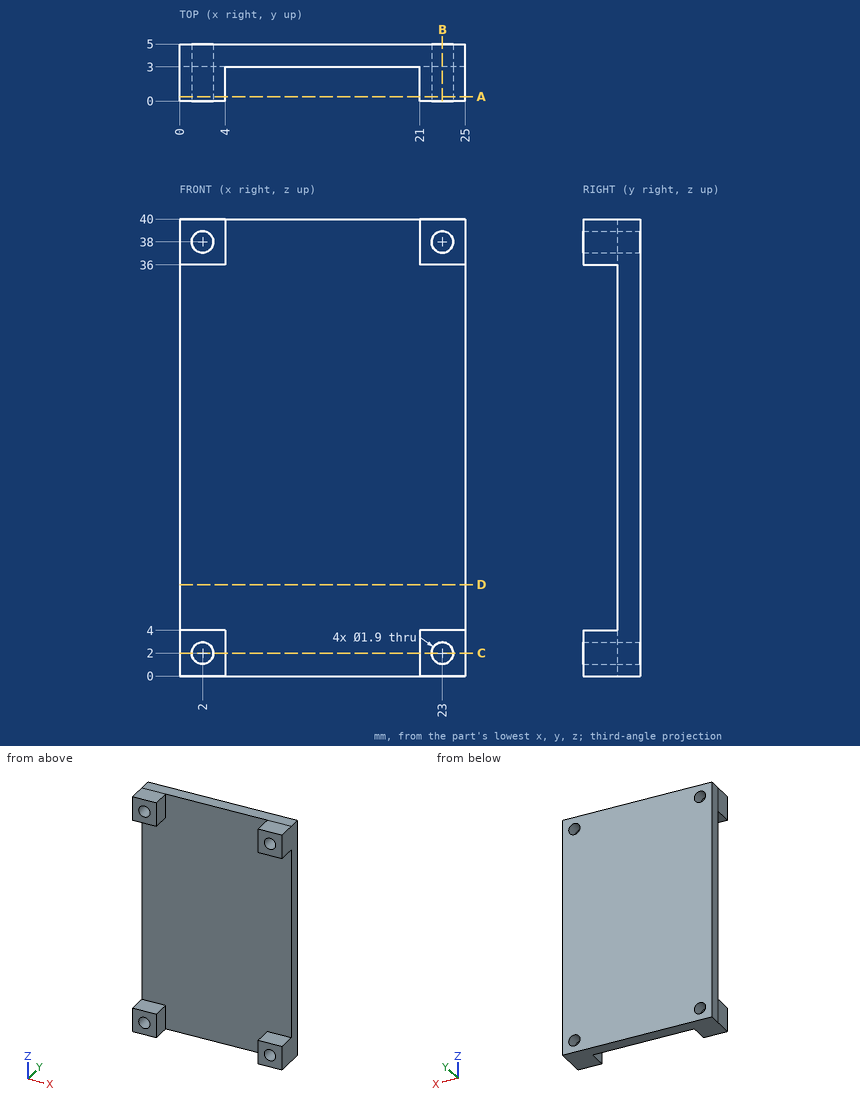
Job drawing, mm, ordinate dimensions from the low corner. One solid piece. Coordinates: 2 decimals unless noted, no trailing zeros. Order: outer loops, then holes, each group sorted by start corner. A loop starts at its lowest first (then second) coordinate and runs counter-clockwise, first axis right, second up. Notation, with made-up numbers: M -36.75,-16.75 L 0.25,-16.75 A24 cw 0.25,5.25 Z; hole C 53,49.5 d10. An arc over 180 degrees is marked long. One line per question, with ' | ' between items.
Q1. Pin check, flat tip, straight feed: P1, Ø7.5, axis at x = 10, z = 17, coming from the -Y side. Stop position of the tip, or through.
A:
P1: stops at y = 3
Q2. Slice it at B-B (x = 23). Give the cut face in (y, z), and give its area (3 significant figures).
A:
outline: M 0,0 L 5,0 L 5,1.05 L 0,1.05 Z; M 0,2.95 L 5,2.95 L 5,37.05 L 0,37.05 L 0,36 L 3,36 L 3,4 L 0,4 Z; M 0,38.95 L 5,38.95 L 5,40 L 0,40 Z | area: 85.0 mm^2
Q3. Slice it at D-D (z = 8). Give the cut face in (x, y).
A:
outline: M 0,3 L 25,3 L 25,5 L 0,5 Z
Q4. Drill centre lines: line 1 (X direction, y = 3.5, z = 2); line 2 (Z direction, x = 23, y = 0.9); line 3 (Y direction, x = 8.75, z = 11). Where is each one in solid material? Low to high.
A:
line 1: x = 0 to 1.05, 2.95 to 22.05, 23.95 to 25 | line 2: z = 0 to 1.05, 2.95 to 4, 36 to 37.05, 38.95 to 40 | line 3: y = 3 to 5
Q5. Slice it at A-A (y = 0.4). Give the cut face in (x, z), and give its area (3 significant figures).
A:
outline: M 0,0 L 4,0 L 4,4 L 0,4 Z; M 0,36 L 4,36 L 4,40 L 0,40 Z; M 21,0 L 25,0 L 25,4 L 21,4 Z; M 21,36 L 25,36 L 25,40 L 21,40 Z; hole C 2,2 d1.9; hole C 2,38 d1.9; hole C 23,2 d1.9; hole C 23,38 d1.9 | area: 52.7 mm^2
Q6. Slice it at C-C (z = 2). Give the cut face in (x, y).
A:
outline: M 0,0 L 1.05,0 L 1.05,5 L 0,5 Z; M 2.95,0 L 4,0 L 4,3 L 21,3 L 21,0 L 22.05,0 L 22.05,5 L 2.95,5 Z; M 23.95,0 L 25,0 L 25,5 L 23.95,5 Z
